Here's how the part is built. I have some questions about the finished solid (model axes, mm). A direction names the side the tool comes from. Coordinates: 2 decimals unless noted, no trailing zeros. Write each loop counter-clockwise with the first axis right and the second up, starting at its lowest first coordinate (ties: lowest second). Pieces come first, ordered by that corner, then holes.
Item 1: Please list where these lines run through material, in increasing order: line 1 (Y direction, x = 0, z = -1.1) (3 decimals); line 2 (Y direction, x = 0, z = 0.8); line 3 (X direction, y = -1, z = -0.3).
Item 2: I'm going to push flat-ended pins straight in: P1, Ø8, axis at x = 13.5, y = 0, coming from the -Z side; P2, Ø2, axis at x = -13.5, y = 1, coming from the -Z side; P3, Ø1, axis at x = 4.5, z = 0, coming from the -Y side. Where does each tip first touch, or does it pass through?
Item 3: If we mould it in two halves opening along Y, with no side actions, what happens to faces 3 (the face through (-17.95, 10.27, -0.02)), 4 (the face through (0.119, -17.462, -0.022)), 5 (the face through (-14.274, -0.628, 0.783))? For each: pulls with the +Y half, pulls with the -Y half, needs draft (parallel to the pull), parting line crosses it, or undercut.
Item 4: For faces 1 (the face through (-31, 0, 0)), 2 (the face through (-11.83, 8.31, 0)), which set-ups out of +Z, -Z, +X, -X, +Y, -Y let a thin tool reach every point of the face, with its end or its side?
Item 5: I want a section at C-C (y = -1.5). Please give me the cut outline in (x, z), and give its area (3 significant figures).
Item 6: I want a section at D-D (y = -9.5). Please give me the cut outline in (x, z).
Item 7: I want a section at A-A (x = 0). Please give me the cut outline in (y, z) (1 decimal).
Item 8: I want a section at B-B (z = -1.1). Count the separate pieces of the cut face and the enclosed holes in it, and give its area (3 significant figures).
Autodesk Inventor part; units mm, degrees
ref_plane "YZ Plane" through (0, 0, 0) normal (1, 0, 0) x (0, 1, 0)
ref_plane "XZ Plane" through (0, 0, 0) normal (0, 1, 0) x (-1, 0, 0)
ref_plane "XY Plane" through (0, 0, 0) normal (0, 0, 1) x (1, 0, 0)
sketch "Sketch1" plane through (0, 0, 0) normal (0, 0, 1) x (1, 0, 0)
  circle A0 centre (0, 0) radius 14.2875
  circle A1 centre (0, 0) radius 15.875
  line L0 (-28.0155, -4.9525) -> (-8.155, -15.4413)
  line L1 (28.0155, -4.9525) -> (8.155, -15.4413)
  line L2 (-8.155, 15.4413) -> (-28.0155, 4.9525)
  line L3 (8.155, 15.4413) -> (28.0155, 4.9525)
  arc A2 (8.155, 15.4413) -> (-8.155, 15.4413) centre (0, 0) ccw
  arc A3 (-8.155, -15.4413) -> (8.155, -15.4413) centre (0, 0) ccw
  arc A4 (-28.0155, 4.9525) -> (-28.0155, -4.9525) centre (-25.4, 0) ccw
  arc A5 (28.0155, -4.9525) -> (28.0155, 4.9525) centre (25.4, 0) ccw
  circle A6 centre (-25.4, 0) radius 2.4892
  circle A7 centre (25.4, 0) radius 2.4892
  dimension "d0" = 28.575
  dimension "d2" = 31.75
  dimension "d3" = 34.925
  dimension "d4" = 4.9784
  dimension "d5" = 50.8
  dimension "d6" = 11.2014
extrude "Extrusion1" add sketch "Sketch1" along normal mid plane 3.175 contours A1 | A4 L2 A2 L3 A5 L1 A3 L0
extrude "Extrusion2" cut sketch "Sketch1" against normal blind 1.5875 contours A1
properties part number "Thriftybot Bearing Hat (TTB-0059)" material "Aluminum 6061"
Answer:
1. line 1: y = -17.462 to -15.875, 15.875 to 17.462
1. line 2: y = -17.46 to -14.29, 14.29 to 17.46
1. line 3: x = -30.91 to -27.68, -23.12 to -15.84, 15.84 to 23.12, 27.68 to 30.91
2. P1: stops at z = -1.59
2. P2: stops at z = 0
2. P3: stops at y = -17
3. face 3: pulls with the +Y half
3. face 4: pulls with the -Y half
3. face 5: undercut
4. face 1: +Z, -Z, -X
4. face 2: -Z
5. outline: (-30.8, -1.59) - (-27.39, -1.59) - (-27.39, 1.59) - (-30.8, 1.59) - close; (-23.41, -1.59) - (-15.8, -1.59) - (-15.8, 0) - (-14.21, 0) - (-14.21, 1.59) - (-23.41, 1.59) - close; (14.21, 0) - (15.8, 0) - (15.8, -1.59) - (23.41, -1.59) - (23.41, 1.59) - (14.21, 1.59) - close; (27.39, -1.59) - (30.8, -1.59) - (30.8, 1.59) - (27.39, 1.59) - close
5. area: 75.0 mm2
6. outline: (-19.4, -1.59) - (-12.72, -1.59) - (-12.72, 0) - (-10.67, 0) - (-10.67, 1.59) - (-19.4, 1.59) - close; (10.67, 0) - (12.72, 0) - (12.72, -1.59) - (19.4, -1.59) - (19.4, 1.59) - (10.67, 1.59) - close
7. outline: (-17.5, -1.6) - (-15.9, -1.6) - (-15.9, 0) - (-14.3, 0) - (-14.3, 1.6) - (-17.5, 1.6) - close; (14.3, 0) - (15.9, 0) - (15.9, -1.6) - (17.5, -1.6) - (17.5, 1.6) - (14.3, 1.6) - close
8. separate pieces: 1
8. enclosed holes: 3
8. area: 570 mm2
